from build123d import *

# Parameters (mm, degrees)
SKETCH_1_R          = 25.5
SKETCH_1_R_2        = 20
EXTRUDE_1_DEPTH     = 6.5
CHAMFER_1_SIZE      = 1.5
CHAMFER_2_SIZE      = 1.5
SKETCH_2_R          = 23.4
SKETCH_2_R_2        = 20.6
CUT_EXTRUDE_1_DEPTH = 0.5
SKETCH_3_R          = 24.9
SKETCH_3_R_2        = 22.1
CUT_EXTRUDE_2_DEPTH = 0.5


with BuildPart() as part:
    # 草图1 → 凸台-拉伸1 (new body)
    with BuildSketch(Plane(origin=(0, 0, 0), x_dir=(1, 0, 0), z_dir=(0, 1, 0))):
        with Locations(Location((0, 0, 0), (0, 0, 90))):
            Circle(SKETCH_1_R)
        with Locations(Location((0, 0, 0), (0, 0, 90))):
            Circle(SKETCH_1_R_2, mode=Mode.SUBTRACT)
    extrude(amount=EXTRUDE_1_DEPTH)

    # 倒角1
    chamfer_1_edges = [part.edges().sort_by_distance(p)[0] for p in [
        (0, 6.5, 25.5),
    ]]
    chamfer(chamfer_1_edges, length=CHAMFER_1_SIZE)

    # 倒角2
    chamfer_2_edges = [part.edges().sort_by_distance(p)[0] for p in [
        (0, 0, 20),
    ]]
    chamfer(chamfer_2_edges, length=CHAMFER_2_SIZE)

    # 草图2 → 切除-拉伸1 (cut)
    with BuildSketch(Plane(origin=(0, 6.5, 0), x_dir=(1, 0, 0), z_dir=(0, 1, 0))):
        with Locations(Location((0, 0, 0), (0, 0, 270))):
            Circle(SKETCH_2_R)
        with Locations(Location((0, 0, 0), (0, 0, 270))):
            Circle(SKETCH_2_R_2, mode=Mode.SUBTRACT)
    extrude(amount=-CUT_EXTRUDE_1_DEPTH, mode=Mode.SUBTRACT)

    # 草图3 → 切除-拉伸2 (cut)
    with BuildSketch(Plane.XZ):
        with Locations(Location((0, 0, 0), (0, 0, 270))):
            Circle(SKETCH_3_R)
        with Locations(Location((0, 0, 0), (0, 0, 270))):
            Circle(SKETCH_3_R_2, mode=Mode.SUBTRACT)
    extrude(amount=-CUT_EXTRUDE_2_DEPTH, mode=Mode.SUBTRACT)


solid = part.part
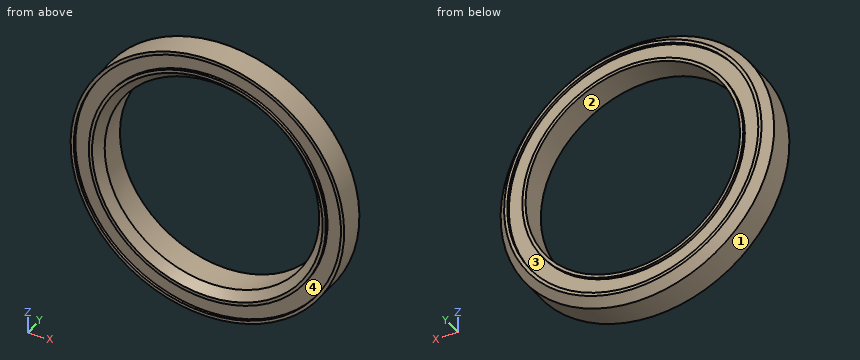
The listing builds one solid part. Answer for the finished solid, in the listing's coordinates (mm). Face numbers are marked on the shaded views. A direction names the side the tool comes from. Give positions to 0.01 mm unless a question says otherwise; leave off trailing zeros. Loops run counter-clockwise (first coordinate to the right, second up) from the corner with the lowest first, then second, coordinate; pieces in that order, holes last.
Item 1: A tool of negligible diameter and unlimited length cuts with its end or side. For the marked faces 3 and 4, from which of +Z, -Z, +X, -X, +Y, -Y can it reach the whole face along a straight path? Write none if from no direction.
Derived:
face 3: +Y
face 4: -Y
Item 2: Each of these flat-tipped pins is pushed along its axis until it touches: pin 1 Ø1.5 at (y, z) = (4.5, 4.5) entering from -X; pin 2 Ø2 at (x, y) = (12, 4.5) entering from +Z; pin 3 Ø15 at (x, z) = (-5, -5.5) entering from -Y; pin 4 Ø1.5 at (x, y) = (-2, 5.5) entering from -Z. Where does it stop, or does it pass through?
Derived:
pin 1: stops at x = -25.22
pin 2: stops at z = 23.01
pin 3: passes through
pin 4: stops at z = -25.46
Item 3: Find the intervals of material crossed by line 1 along X through (y, z) = (6.1, 0); line 2 along X through (y, z) = (6.3, 0); line 3 along X through (y, z) = (1.75, 4), in increasing order.
Derived:
line 1: x = -24.4 to -23.4, -20.6 to -20, 20 to 20.6, 23.4 to 24.4
line 2: x = -24.2 to -23.4, -20.6 to -20, 20 to 20.6, 23.4 to 24.2
line 3: x = -25.18 to -19.6, 19.6 to 25.18
Item 4: Determine the mould class of the marked faces 1 and 2 for opening direction X: +X half, -X half, draft (parallel to the pull), parting line (faces both ways), or undercut.
Derived:
face 1: parting line
face 2: undercut
Item 5: A cutting plane is placed at A-A (z = 0). Give the vertices of the cut face in (x, y), then the cut area to 3 significant figures.
Derived:
outline: (-25.5, 0) - (-24.9, 0) - (-24.9, 0.5) - (-22.1, 0.5) - (-22.1, 0) - (-21.5, 0) - (-20, 1.5) - (-20, 6.5) - (-20.6, 6.5) - (-20.6, 6) - (-23.4, 6) - (-23.4, 6.5) - (-24, 6.5) - (-25.5, 5) - close; (20, 1.5) - (21.5, 0) - (22.1, 0) - (22.1, 0.5) - (24.9, 0.5) - (24.9, 0) - (25.5, 0) - (25.5, 5) - (24, 6.5) - (23.4, 6.5) - (23.4, 6) - (20.6, 6) - (20.6, 6.5) - (20, 6.5) - close
area: 61.4 mm2
Item 6: A cutting plane is placed at C-C (y = 3). Give the vertices of the cut face in (x, z).
Derived:
outline: circle Ø51 at (0, 0); hole circle Ø40 at (0, 0)
Item 7: A cutting plane is placed at B-B (x = 0). Give the vertices of the cut face in (y, z), then the cut area to 3 significant figures.
Derived:
outline: (0, -25.5) - (5, -25.5) - (6.5, -24) - (6.5, -23.4) - (6, -23.4) - (6, -20.6) - (6.5, -20.6) - (6.5, -20) - (1.5, -20) - (0, -21.5) - (0, -22.1) - (0.5, -22.1) - (0.5, -24.9) - (0, -24.9) - close; (0, 21.5) - (1.5, 20) - (6.5, 20) - (6.5, 20.6) - (6, 20.6) - (6, 23.4) - (6.5, 23.4) - (6.5, 24) - (5, 25.5) - (0, 25.5) - (0, 24.9) - (0.5, 24.9) - (0.5, 22.1) - (0, 22.1) - close
area: 61.4 mm2
